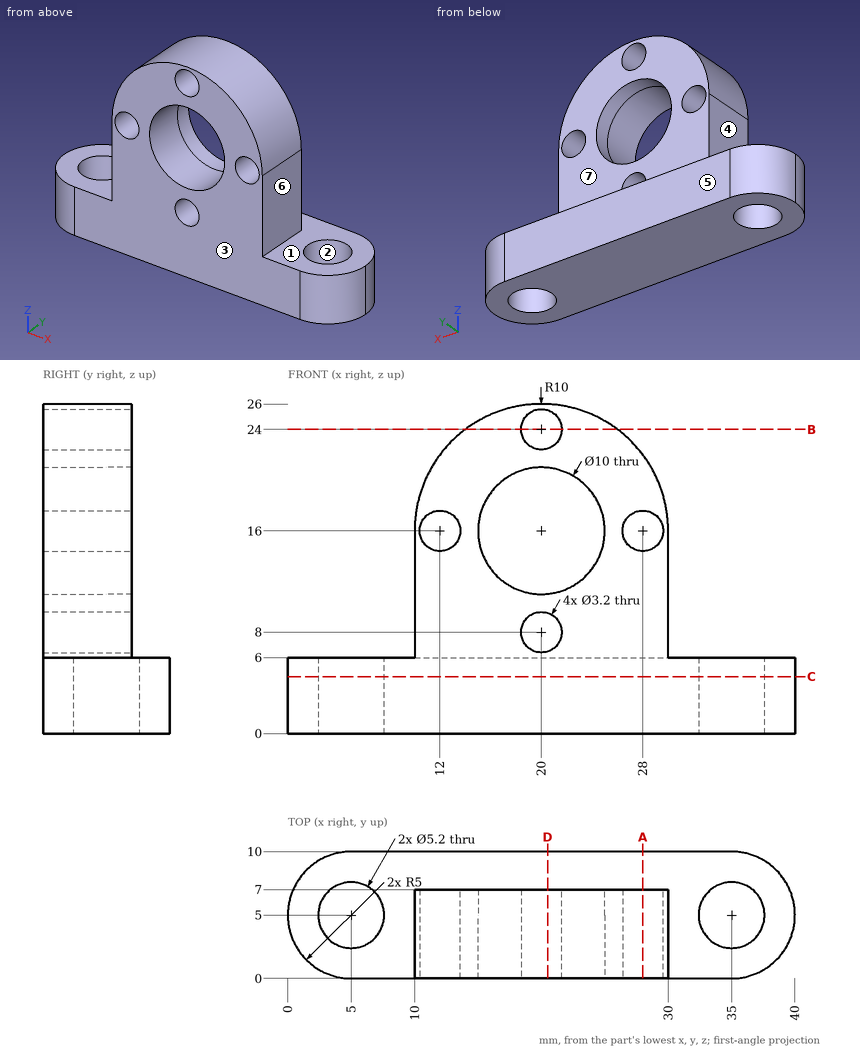
Here's the drawing with two shaded views (mm, measured from the low corner). I have some questions. A direction names the side the tool comes from. Round coordinates to 2 decimals unless told otherwise and drop trailing zeros. Loops run counter-clockwise (first coordinate to the right, second up) from the corner with the lowest first, then second, coordinate; pieces in that order, holes last.
1. Suppose I cut it at C-C, the plane z = 4.5. Please give me the cut outline in (x, y), and give its area (3 significant figures).
Answers:
outline: (5, 0) - (35, 0) arc R5 ccw to (35, 10) - (5, 10) arc R5 ccw to start; hole circle Ø5.2 at (5, 5); hole circle Ø5.2 at (35, 5)
area: 336 mm2
2. Suppose I cut it at A-A, the plane x = 28. Please give me the cut outline in (y, z), and give its area (3 significant figures).
Answers:
outline: (0, 0) - (10, 0) - (10, 6) - (7, 6) - (7, 14.4) - (0, 14.4) - close; (0, 17.6) - (7, 17.6) - (7, 22) - (0, 22) - close
area: 150 mm2
3. Will these pins go through, and if not, where does the flat tip stop? pin 1 (2 mm diameter, centred on y = 2, z = 13, fed in from +X); pin 2 (5 mm diameter, centred on x = 12, z = 16, fed in from +Y); pin 3 (3 mm diameter, centred on y = 1.5, z = 4, fed in from +X); pin 4 (1 mm diameter, centred on x = 29, z = 16, fed in from -Y).
Answers:
pin 1: stops at x = 30
pin 2: stops at y = 7
pin 3: stops at x = 39.58
pin 4: passes through
4. Suppose I cut it at B-B, the plane z = 24. Please give me the cut outline in (x, y).
Answers:
outline: (14, 0) - (18.4, 0) - (18.4, 7) - (14, 7) - close; (21.6, 0) - (26, 0) - (26, 7) - (21.6, 7) - close
5. If I drill on probe 1 along Z at (x, y) = (20, 4); probe 2 along Y at (x, z) = (15.5, 20); probe 3 along X at (y, z) = (1, 12), over which ranges is the centre line in solid material (lowest first)?
Answers:
probe 1: z = 0 to 6.4, 9.6 to 11, 21 to 22.4, 25.6 to 26
probe 2: y = 0 to 7
probe 3: x = 10 to 17, 23 to 30
6. For the marked faces 4, 5, 6 and 7, which set-ups out of +Z, -Z, +X, -X, +Y, -Y let a thin tool reach every point of the face, with its end or its side?
Answers:
face 4: +Z, -X, +Y, -Y
face 5: +Z, -Z, +X, -X, +Y
face 6: +Z, +X, +Y, -Y
face 7: +Z, +X, -X, +Y
7. Suppose I cut it at D-D, the plane x = 20.5. Please give me the cut outline in (y, z), and give its area (3 significant figures).
Answers:
outline: (0, 0) - (10, 0) - (10, 6) - (7, 6) - (7, 6.48) - (0, 6.48) - close; (0, 9.52) - (7, 9.52) - (7, 11.03) - (0, 11.03) - close; (0, 20.97) - (7, 20.97) - (7, 22.48) - (0, 22.48) - close; (0, 25.52) - (7, 25.52) - (7, 25.99) - (0, 25.99) - close
area: 87.7 mm2
8. Thinking about a two-plate mould opening in Y: for the marked faces 1, 2 and 3, which applies, released by +Y, released by -Y, zero draft, split by the parting line, or undercut?
Answers:
face 1: zero draft
face 2: undercut
face 3: released by -Y
